Build history of the part. All positions in model axes, mm. A direction names the side the tool comes from. Round coordinates to 2 decimals unless told otherwise and drop trailing zeros. Write each loop counter-clockwise with the first axis right and the second up, starting at its lowest first coordinate (ties: lowest second). Pieces come first, ordered by that corner, then holes. Notation, with made-up numbers: M 15,27.5 L 36,27.5 A19 cw 36,49.5 Z; hole C 6,29.25 d3. An arc over 180 degrees is marked long. Use a Markdown table: item, result.
from build123d import *

# Parameters (mm, degrees)
SKETCH1_R           = 9
SKETCH1_R_2         = 4
SKETCH1_R_3         = 14
BOSS_EXTRUDE1_DEPTH = 10
BOSS_EXTRUDE2_DEPTH = 1


with BuildPart() as part:
    # Sketch1 → Boss-Extrude1 (new body)
    with BuildSketch(Plane.XY):
        with BuildLine():
            Line((-22, -54), (-41.469262149, -54))
            ThreePointArc((-41.469262149, -54), (-58.686185522, -68.620791716), (-48.072286471, -88.559075187))
            ThreePointArc((-48.072286471, -88.559075187), (-43.655027403, -92.245315871), (-42, -97.755436773))
            Line((-42, -97.755436773), (-42, -102))
            Line((-42, -102), (42, -102))
            Line((42, -102), (42, -97.748786379))
            ThreePointArc((42, -97.748786379), (43.654770396, -92.239054729), (48.071428571, -88.552791244))
            ThreePointArc((48.071428571, -88.552791244), (56.944278467, -80.353441457), (58.634486701, -68.391000304))
            Line((58.634486701, -68.391000304), (57.453450889, -64.700414132))
            ThreePointArc((57.453450889, -64.700414132), (50.813446244, -56.910391893), (41, -54))
            Line((41, -54), (22, -54))
            ThreePointArc((22, -54), (16.343145751, -51.656854249), (14, -46))
            Line((14, -46), (14, -33.255572853))
            ThreePointArc((14, -33.255572853), (15.413257736, -31.731290406), (17.111111111, -30.532112219))
            ThreePointArc((17.111111111, -30.532112219), (0, 35), (-17.111111111, -30.532112219))
            ThreePointArc((-17.111111111, -30.532112219), (-15.413257736, -31.731290406), (-14, -33.255572853))
            Line((-14, -33.255572853), (-14, -46))
            ThreePointArc((-14, -46), (-16.343145751, -51.656854249), (-22, -54))
        make_face()
        with Locations((-41, -72)):
            Circle(SKETCH1_R, mode=Mode.SUBTRACT)
        with Locations((41, -72)):
            Circle(SKETCH1_R, mode=Mode.SUBTRACT)
        with Locations((12, 20.784609691)):
            Circle(SKETCH1_R_2, mode=Mode.SUBTRACT)
        with Locations((-12, -20.784609691)):
            Circle(SKETCH1_R_2, mode=Mode.SUBTRACT)
        with Locations((-24, 0)):
            Circle(SKETCH1_R_2, mode=Mode.SUBTRACT)
        with Locations((-12, 20.784609691)):
            Circle(SKETCH1_R_2, mode=Mode.SUBTRACT)
        with Locations((12, -20.784609691)):
            Circle(SKETCH1_R_2, mode=Mode.SUBTRACT)
        Circle(SKETCH1_R_3, mode=Mode.SUBTRACT)
        with Locations((24, 0)):
            Circle(SKETCH1_R_2, mode=Mode.SUBTRACT)
    extrude(amount=BOSS_EXTRUDE1_DEPTH)

    # Sketch1_3 → Boss-Extrude2 (add)
    with BuildSketch(Plane.XY):
        with BuildLine():
            Line((57.453450889, -64.700414132), (33.334718679, 10.667545668))
            ThreePointArc((33.334718679, 10.667545668), (34.581173735, 5.398372265), (35, 0))
            ThreePointArc((35, 0), (30.198417913, -17.693376036), (17.111111111, -30.532112219))
            ThreePointArc((17.111111111, -30.532112219), (15.413257736, -31.731290406), (14, -33.255572853))
            Line((14, -33.255572853), (14, -46))
            ThreePointArc((14, -46), (16.343145751, -51.656854249), (22, -54))
            Line((22, -54), (41, -54))
            ThreePointArc((41, -54), (50.813446244, -56.910391893), (57.453450889, -64.700414132))
        make_face()
        with BuildLine():
            ThreePointArc((-58.141884058, -66.488555733), (-51.79486562, -57.58850864), (-41.469262149, -54))
            Line((-41.469262149, -54), (-22, -54))
            ThreePointArc((-22, -54), (-16.343145751, -51.656854249), (-14, -46))
            Line((-14, -46), (-14, -33.255572853))
            ThreePointArc((-14, -33.255572853), (-15.413257736, -31.731290406), (-17.111111111, -30.532112219))
            ThreePointArc((-17.111111111, -30.532112219), (-32.56606191, -12.823868827), (-33.334718679, 10.667545668))
            Line((-33.334718679, 10.667545668), (-58.141884058, -66.488555733))
        make_face()
    extrude(amount=BOSS_EXTRUDE2_DEPTH)


solid = part.part
Q1. Drop flat-ended pins along their axis: P1, Ø1, axis at y = -56.5, z = 8, coming from the -X side; P2, Ø25, axis at x = 0, y = 0, coming from the -Z side; P3, Ø2.5, axis at y = -40.5, z = 7, coming from the +X side; P4, Ø4.5, axis at y = -101, z = 3.5, coming from the +X side. Give the stop position or say it passes through.
Response values:
| item | result |
|---|---|
| P1 | stops at x = -50.96 |
| P2 | passes through |
| P3 | stops at x = 14 |
| P4 | stops at x = 42 |
Q2. Cut at A-A on x = 0. Give the cut face in (y, z).
Response values:
| item | result |
|---|---|
| outline | M -102,0 L -14,0 L -14,10 L -102,10 Z; M 14,0 L 35,0 L 35,10 L 14,10 Z |
Q3. Cut at D-D on z = 3.75. Count the separate pieces of the cut face and the enclosed holes in it, and give its area (3 significant figures).
Response values:
| item | result |
|---|---|
| separate pieces | 1 |
| enclosed holes | 9 |
| area | 8,010 mm2 |
Q4. Two-plate mould, pull along X, no slides. Class faces 5 (the cylindrical face through (-58.62, -68.29, 4.93)), 6 (the cylindrical face through (-27.2, -2.4, 4.9)), 7 (the flat face through (-32, -54, 5)): +X half, -X half, draft (parallel to the pull), parting line (faces both ways), or undercut.
Response values:
| item | result |
|---|---|
| face 5 | -X half |
| face 6 | undercut |
| face 7 | draft |
Q5. Drill centre lines: L1, parallel to Y at x = 24, z = 7.75; L2, parallel to Y at x = 15, z = 1.25; L3, parallel to Y at x = -1, z = 9. Where is each one in solid material? Low to high.
Response values:
| item | result |
|---|---|
| L1 | y = -102 to -54, -25.48 to -4, 4 to 25.48 |
| L2 | y = -102 to -49.87, -32.11 to -23.43, -18.14 to 18.14, 23.43 to 31.62 |
| L3 | y = -102 to -13.96, 13.96 to 34.99 |
Q6. Cut at C-C on y = -75. Give the cut face in (x, z), and give its area (3 significant figures).
Response values:
| item | result |
|---|---|
| outline | M -58.75,0 L -49.49,0 L -49.49,10 L -58.75,10 Z; M -32.51,0 L 32.51,0 L 32.51,10 L -32.51,10 Z; M 49.49,0 L 58.75,0 L 58.75,10 L 49.49,10 Z |
| area | 836 mm2 |
Q7. Cut at B-B on y = -8.5. Give the cut face in (x, z).
Response values:
| item | result |
|---|---|
| outline | M -39.5,0 L -11.12,0 L -11.12,10 L -33.95,10 L -33.95,1 L -39.5,1 Z; M 11.12,0 L 39.47,0 L 39.47,1 L 33.95,1 L 33.95,10 L 11.12,10 Z |
Q8. Which spindle directions (+Z, -Z, +X, -X, +Y, -Y) get a long thin tool onto all of the face, cutting with end or side? Do faces 1 (the cylindrical face through (50.935, -56.99, 5.437)), 2 (the flat face through (32, -54, 5)), 3 (the cylindrical face through (1.289, 34.976, 4.93)), 4 (the flat face through (-14, -40, 5)). Say none if no direction does.
Response values:
| item | result |
|---|---|
| face 1 | +Z, +X, +Y |
| face 2 | +Z, +X |
| face 3 | +Z |
| face 4 | +Z, -X |
